from build123d import *


with BuildPart() as part:
    # Sketch1 → Revolve1 (revolve)
    with BuildSketch(Plane.XY):
        Polygon((0, 0), (0, 3.57505), (0.508, 4.08305), (2.9083, 4.08305), (3.4671, 3.52425), (4.0259, 3.52425), (4.0259, 4.5593), (7.8232, 4.5593), (8.3312, 4.0513), (8.3312, 0), align=None)
    revolve(axis=Axis((8.3312, 0, 0), (-1, 0, 0)))

    # Sketch2 → Cut-Revolve1 (revolve, cut)
    with BuildSketch(Plane.XY):
        Polygon((0, 0), (0, 2.413), (0.42926, 1.98374), (7.90194, 1.98374), (8.3312, 2.413), (8.3312, 0), align=None)
    revolve(axis=Axis((8.3312, 0, 0), (-1, 0, 0)), mode=Mode.SUBTRACT)

    # Sketch3 → Revolve2 (revolve)
    with BuildSketch(Plane.XY):
        with BuildLine():
            Line((3.306480735, 4.475131804), (3.912128708, 3.869483831))
            ThreePointArc((3.912128708, 3.869483831), (3.949326147, 3.779681269), (3.912128708, 3.689878708))
            Line((3.912128708, 3.689878708), (3.7465, 3.52425))
            Line((3.7465, 3.52425), (3.4671, 3.52425))
            Line((3.4671, 3.52425), (3.4671, 3.27025))
            Line((3.4671, 3.27025), (4.0259, 3.27025))
            Line((4.0259, 3.27025), (4.0259, 4.043080735))
            Line((4.0259, 4.043080735), (3.509680735, 4.5593))
            Line((3.509680735, 4.5593), (3.306480735, 4.5593))
            Line((3.306480735, 4.5593), (3.306480735, 4.475131804))
        make_face()
    revolve(axis=Axis((4.0259, 0, 0), (-1, 0, 0)))


solid = part.part
Design review of the part built by this model. Coordinates are the model's own, in mm. Round coordinates to 2 decimals unless told otherwise and drop trailing zeros. Write each loop counter-clockwise with the first axis right and the second up, starting at its lowest first coordinate (ties: lowest second). Pieces come first, ordered by that corner, then holes. Notation, with made-up numbers: M -39.75,10 L -16.75,10 A21 cw -16.75,27 Z; hole C -34,19 d9. An arc over 180 degrees is marked long. One line per item, written item: value. Start each with the question number.
1. Clearance check with flat-ended pins moving along their axes: P1, Ø3.5, axis at y = 0, z = 0, coming from the +X side; P2, Ø1.5, axis at x = 2, z = -1, coming from the +Y side; P3, Ø3, axis at x = 4, z = 3, coming from the +Y side. State where each tip first meets the part, or that it passes through.
2. To check wall thickness, follow probe 1 along Y at (x, z) = (4.5, 0); probe 2 along Z at (x, y) = (2.5, 0). State the ranges of each line that lie inside material, in increasing order. Write a range as from..to.
3. Take a section at A-A on x = 7.5. State the section outline as (y, z) points.
4. Draft analysis for pull direction Y (two halves, no side actions). For faces 1 (the face through (4.218, -0.258, -1.967)), 2 (the face through (8.331, 2, 2)), 3 (the face through (6, -3.6, 2.8)), state which applies: pulls with the +Y half, pulls with the -Y half, needs draft (parallel to the pull), parting line crosses it, or undercut.
Computed:
1. P1: passes through
1. P2: stops at y = 4.08
1. P3: stops at y = 4.31
2. probe 1: y = -4.56..-1.98, 1.98..4.56
2. probe 2: z = -4.08..-1.98, 1.98..4.08
3. outline: C 0,0 d9.12; hole C 0,0 d3.97
4. face 1: undercut
4. face 2: needs draft
4. face 3: parting line crosses it
